```python
from build123d import *

# Parameters (mm, degrees)
BOSS_EXTRUDE1_DEPTH     = 2.5
CUT_EXTRUDE1_DEPTH      = 107.279407695
CUT_EXTRUDE2_DEPTH      = 107.191160178
CUT_EXTRUDE2_DEPTH_BACK = 107.191160178
SKETCH6_R               = 1.375


with BuildPart() as part:
    # Sketch3 → Boss-Extrude1 (new, symmetric)
    with BuildSketch(Plane.XY):
        with BuildLine():
            ThreePointArc((5.967243679, 21.694285028), (-22.5, 0), (5.967243679, -21.694285028))
            ThreePointArc((5.967243679, -21.694285028), (52.625175797, -10.843791309), (100, -3.75))
            ThreePointArc((100, -3.75), (103.75, 0), (100, 3.75))
            ThreePointArc((100, 3.75), (52.625175797, 10.843791309), (5.967243679, 21.694285028))
        make_face()
        with BuildLine():
            Line((-18.9, -7.5), (18.9, -7.5))
            ThreePointArc((18.9, -7.5), (0, -20.333715843), (-18.9, -7.5))
        make_face(mode=Mode.SUBTRACT)
        with BuildLine():
            Line((-18.9, 7.5), (18.9, 7.5))
            ThreePointArc((18.9, 7.5), (0, 20.333715843), (-18.9, 7.5))
        make_face(mode=Mode.SUBTRACT)
        with BuildLine():
            ThreePointArc((15.104191038, 16.676732686), (55.600003106, 7.741362472), (96.614544634, 1.612821119))
            ThreePointArc((96.614544634, 1.612821119), (96.25, 0), (96.614544634, -1.612821119))
            ThreePointArc((96.614544634, -1.612821119), (55.600003106, -7.741362472), (15.104191038, -16.676732686))
            ThreePointArc((15.104191038, -16.676732686), (22.5, 0), (15.104191038, 16.676732686))
        make_face(mode=Mode.SUBTRACT)
    extrude(amount=BOSS_EXTRUDE1_DEPTH, both=True)

    # Sketch4 → Cut-Extrude1 (cut, through all)
    with BuildSketch(Plane.XY.offset(2.5)):
        with BuildLine():
            Line((-16.97242536, 2.514767746), (-3.665719575, 4.75))
            ThreePointArc((-3.665719575, 4.75), (0, 6), (3.665719575, 4.75))
            Line((3.665719575, 4.75), (16.97242536, 2.514767746))
            ThreePointArc((16.97242536, 2.514767746), (19.1, 0), (16.97242536, -2.514767746))
            Line((16.97242536, -2.514767746), (3.665719575, -4.75))
            ThreePointArc((3.665719575, -4.75), (0, -6), (-3.665719575, -4.75))
            Line((-3.665719575, -4.75), (-16.97242536, -2.514767746))
            ThreePointArc((-16.97242536, -2.514767746), (-19.1, 0), (-16.97242536, 2.514767746))
        make_face()
    extrude(amount=-CUT_EXTRUDE1_DEPTH, mode=Mode.SUBTRACT)

    # Sketch6 → Cut-Extrude2 (cut, two sides: drawn at the far end of the back side and taken through both)
    with BuildSketch(Plane.XY.offset(-CUT_EXTRUDE2_DEPTH_BACK)):
        with Locations((100, 0)):
            Circle(SKETCH6_R)
    extrude(amount=CUT_EXTRUDE2_DEPTH + CUT_EXTRUDE2_DEPTH_BACK, mode=Mode.SUBTRACT)


solid = part.part
```
Verification items for the finished model (mm, model axes). A direction names the side the tool comes from. Give positions to 0.01 mm unless a question says otherwise; leave off trailing zeros. Order: outer loops, then holes, each group sorted by start corner. A loop starts at its lowest first (then second) coordinate and runs counter-clockwise, first axis right, second up. Notation, with made-up numbers: M 86.5,33 L 142.5,33 A9 ccw 142.5,39 Z; hole C -26,-24.75 d3. An arc over 180 degrees is marked long. Answer in a Markdown table with one row per item. Add a question column.
Item 1: Section check C-C, the plane y = 0. Enter the section's corners in (x, z) (3 decimals), and give its area (4 significant figures).
Item 2: Section check A-A, the plane x = 0. Enter the section's corners in (y, z).
Item 3: Gauge pin test, flat ends, axial feed: pin 1 (2 mm diameter, centred on x = 91, z = 0, fed in from +Y); pin 2 (3 mm diameter, centred on x = -5, z = 0, fed in from +Y); pin 3 (1 mm diameter, centred on x = 38, z = -2, fed in from -Y). Record the tip position at first contact, or that the pin passes through.
Item 4: Mould release check, pull along X, two halves, no side actions. Record for faces 1 (the cylindrical face through (103.75, -0.08, 0.04)), 2 (the flat face through (22, -2, -2.5)), 3 (the flat face through (10.412, -3.617, 0.035)): released by +X, released by -X, zero draft, split by the parting line, or undercut.
Item 5: Scan lines: probe 1 along X at (y, z) = (0, 0.4) (3 decimals); probe 2 along X at (y, z) = (1.5, 2); probe 3 along Y at (x, z) = (-3, -1.75). Record each from-to range of solid material in increasing order. Write a range as from..to.
Item 6: Section check D-D, the plane x = 33. Enter the section's corners in (y, z), and give its area (3 significant figures).
Item 7: Tool access check on faces 4 (the cylindrical face through (53.28, 10.72, 0.04)), 5 (the cylindrical face through (-19.1, -0.1, 0)). Record the directions out of +Z, -Z, +X, -X, +Y, -Y that give a thin tool (end or side, any length) a straight path to the whole face; none if there is none.
Item 8: Section check B-B, the plane z = -1.25. Enter the section's corners in (x, y) (3 decimals), and give its area (3 significant figures).
Filled sheet:
| question | item | result |
|---|---|---|
| 1 | outline | M -22.5,-2.5 L -19.1,-2.5 L -19.1,2.5 L -22.5,2.5 Z; M 19.1,-2.5 L 22.5,-2.5 L 22.5,2.5 L 19.1,2.5 Z; M 96.25,-2.5 L 98.625,-2.5 L 98.625,2.5 L 96.25,2.5 Z; M 101.375,-2.5 L 103.75,-2.5 L 103.75,2.5 L 101.375,2.5 Z |
| 1 | area | 57.75 mm^2 |
| 2 | outline | M -22.5,-2.5 L -20.33,-2.5 L -20.33,2.5 L -22.5,2.5 Z; M -7.5,-2.5 L -6,-2.5 L -6,2.5 L -7.5,2.5 Z; M 6,-2.5 L 7.5,-2.5 L 7.5,2.5 L 6,2.5 Z; M 20.33,-2.5 L 22.5,-2.5 L 22.5,2.5 L 20.33,2.5 Z |
| 3 | pin 1 | stops at y = 4.93 |
| 3 | pin 2 | stops at y = 22.23 |
| 3 | pin 3 | stops at y = -13.93 |
| 4 | face 1 | released by +X |
| 4 | face 2 | zero draft |
| 4 | face 3 | undercut |
| 5 | probe 1 | x = -22.5..-19.1, 19.1..22.5, 96.25..98.625, 101.375..103.75 |
| 5 | probe 2 | x = -22.45..-18.61, 18.61..22.45, 96.56..103.44 |
| 5 | probe 3 | y = -22.3..-20.11, -7.5..-5.2, 5.2..7.5, 20.11..22.3 |
| 6 | outline | M -14.93,-2.5 L -12.37,-2.5 L -12.37,2.5 L -14.93,2.5 Z; M 12.37,-2.5 L 14.93,-2.5 L 14.93,2.5 L 12.37,2.5 Z |
| 6 | area | 25.6 mm^2 |
| 7 | face 4 | +Z, -Z, +X, +Y |
| 7 | face 5 | +Z, -Z |
| 8 | outline | M 5.967,-21.694 A600 cw 100,-3.75 A3.75 ccw 100,3.75 A600 cw 5.967,21.694 A22.5 ccw long Z; hole M -18.9,-7.5 A20.334 ccw 18.9,-7.5 Z; hole M -18.9,7.5 L 18.9,7.5 A20.334 ccw Z; hole M -16.972,-2.515 L -3.666,-4.75 A6 ccw 3.666,-4.75 L 16.972,-2.515 A2.55 ccw 16.972,2.515 L 3.666,4.75 A6 ccw -3.666,4.75 L -16.972,2.515 A2.55 ccw Z; hole M 15.104,-16.677 A602.5 cw 96.615,-1.613 A3.75 cw 96.615,1.613 A602.5 cw 15.104,16.677 A22.5 cw Z; hole C 100,0 d2.75 |
| 8 | area | 1,070 mm^2 |
